Work out the finished part from the listing and answer in its coordinate system (mm). A direction names the side the tool comes from. Round coordinates to 2 decimals unless told otherwise and drop trailing zeros. Loops run counter-clockwise (first coordinate to the right, second up) from the corner with the lowest first, then second, coordinate; pieces in that order, holes last. Notation, with made-up numbers: M 42.25,11 L 56.25,11 A37 ccw 56.25,48 Z; hole C -35,54.25 d8. An arc over 180 degrees is marked long. One line per item, written item: value.
Autodesk Inventor part; units mm, degrees
ref_plane "YZ Plane" through (0, 0, 0) normal (1, 0, 0) x (0, 1, 0)
ref_plane "XZ Plane" through (0, 0, 0) normal (0, 1, 0) x (-1, 0, 0)
ref_plane "XY Plane" through (0, 0, 0) normal (0, 0, 1) x (1, 0, 0)
sketch "Sketch1" plane through (0, 0, 0) normal (0, 0, 1) x (1, 0, 0)
  line L0 (0, 0) -> (16.25, 0)
  line L1 (44, 0) -> (44, 22)
  line L2 (44, 22) -> (16.25, 22)
  line L3 (0, 22) -> (0, 0)
  line L4 (5.25, 18) -> (10.5, 18)
  line L5 (10.5, 18) -> (10.5, 12.75)
  line L6 (10.5, 12.75) -> (5.25, 12.75)
  line L7 (5.25, 12.75) -> (5.25, 18)
  line L8 (16.25, 22) -> (16.25, 0)
  line L9 (16.25, 22) -> (0, 22)
  line L10 (16.25, 0) -> (44, 0)
  circle A0 centre (21.5, 5.25) radius 2.625
  circle A1 centre (36, 15.25) radius 4.75
  circle A2 centre (36, 15.25) radius 4
  circle A3 centre (36, 15.25) radius 2.625
  dimension "d0" = 44
  dimension "d1" = 22
  dimension "d2" = 5.25
  dimension "d3" = 5.25
  dimension "d4" = 16.25
  dimension "d5" = 5.25
  dimension "d6" = 5.25
  dimension "d7" = 5.25
  dimension "d8" = 4
  dimension "d9" = 5.25
  dimension "d10" = 6.75
  dimension "d11" = 8
  dimension "d12" = 5.25
  dimension "d13" = 8
  dimension "d14" = 9.5
extrude "Extrusion1" add sketch "Sketch1" along normal blind 8 contours L3 L9 L8 L0 | L8 L2 L1 L10 | A1 | A2 | A3
extrude "Extrusion2" add sketch "Sketch1" along normal blind 16.25 contours L3 L9 L8 L0 | A1
extrude "Extrusion3" add sketch "Sketch1" along normal blind 13 contours A2 | A3
chamfer "Chamfer1" distance 3.25 distance2 1.25 1 edges at (32, 15.25, 13) measured on face at (39.987, 14.9281, 15.1667)
1) Find section C-C (z = 3.25). Give the vertices of the cut face in (x, y) (3 decimals), then the cut area to 3 significant figures.
Check values:
outline: M 0,0 L 44,0 L 44,22 L 0,22 Z; hole M 5.25,12.75 L 10.5,12.75 L 10.5,18 L 5.25,18 Z; hole C 21.5,5.25 d5.25
area: 919 mm2
2) Find section A-A (y = 5.25). Give the vertices of the cut face in (x, z) (3 decimals), then the cut area to 3 significant figures.
Check values:
outline: M 0,0 L 18.875,0 L 18.875,8 L 16.25,8 L 16.25,16.25 L 0,16.25 Z; M 24.125,0 L 44,0 L 44,8 L 24.125,8 Z
area: 444 mm2
3) Find section B-B (x = 21.5). Give the vertices of the cut face in (y, z) (3 decimals).
Check values:
outline: M 0,0 L 2.625,0 L 2.625,8 L 0,8 Z; M 7.875,0 L 22,0 L 22,8 L 7.875,8 Z
4) Each of these flat-tipped pins is pushed along its axis until it touches: pin 1 (4 mm diameter, centred on x = 21.5, y = 5.25, fed in from +Z); pin 2 (4 mm diameter, centred on y = 14, z = 10.5, fed in from +X). Where does it stop, or does it pass through?
Check values:
pin 1: through
pin 2: x = 40.75
5) Find the intervals of material crossed by probe 1 along X at (y, z) = (17.5, 13.25); probe 2 along X at (y, z) = (13, 13.5); probe 3 along Y at (x, z) = (8.5, 13.75), in increasing order. Write a range as from..to.
Check values:
probe 1: 0..5.25, 10.5..16.25, 31.82..34.26, 37.74..40.18
probe 2: 0..5.25, 10.5..16.25, 31.82..34.1, 37.9..40.18
probe 3: 0..12.75, 18..22
6) The mould has two halves that part along Y. Classify faces 4 (the face through (8, 12.75, 8)), 5 (the face through (8, 18, 8)), 6 (the face through (17, 22, 6)), 7 (the face through (8, 11, 16.25)): +Y half, -Y half, draft (parallel to the pull), parting line (faces both ways), or undercut.
Check values:
face 4: undercut
face 5: undercut
face 6: +Y half
face 7: draft
7) For faces 1 (the face through (16.25, 11, 12)), 2 (the face through (5.25, 15, 8)), 3 (the face through (36, 15, 13)), determine the directions among +Z, -Z, +X, -X, +Y, -Y from which every point of the face is accessible in a straight line to the end or side of a thin tool.
Check values:
face 1: +Z, +Y, -Y
face 2: +Z, -Z
face 3: +Z
